Here's how the part is built. I have some questions about the finished solid (model axes, mm). Give positions to 0.01 mm unless a question says otherwise; leave off trailing zeros. Loops run counter-clockwise (first coordinate to the right, second up) from the corner with the lowest first, then second, coordinate; pieces in that order, holes last.
Q1. Suppose I cut it at A-A (z = 0). List the corners of the cut face in (x, y) for me (3 decimals), and give its area (3 significant figures).
Q2. Thinking about a two-plate mould opening in Y: for faces 1 (the face through (-7.559, 214.845, 5.796)), 2 (the face through (-4, 0, -4)), which applies, pulls with the +Y half, pulls with the -Y half, needs draft (parallel to the pull), parting line crosses it, or undercut?
Q3. I'm going to push flat-ended pins straight in: P1, Ø12.5, axis at x = 63.5, z = 285.75, coming from the +Y side; P2, Ø8.5, axis at x = -63.5, z = 285.75, coming from the -Y side. Where does each tip first touch, or does it pass through?
Q4. I need wall thicknesses on probe 1 along Z at (x, y) = (63.5, 2.25); probe 2 along Z at (x, y) = (-285.75, 3.25). Which ranges of each line are inside material? Lowest first, please.
Q5. Suppose I cut it at C-C (y = 148). List the corners of the cut face in (x, z) for me (3 decimals).
Q6. Suppose I cut it at B-B (x = 0). List the corners of the cut face in (y, z) for me (3 decimals), and give its area (3 significant figures).
Q7. Suppose I cut it at D-D (z = -262.5). List the corners of the cut face in (x, y) for me.
```python
from build123d import *

# Parameters (mm, degrees)
SKETCH1_W                        = 609.6
SKETCH1_H                        = 609.6
BOSS_EXTRUDE1_DEPTH              = 6.35
F_3_8_0_375_DIAMETER_HOLE1_D     = 9.525
F_3_8_0_375_DIAMETER_HOLE1_DEPTH = 11.684
F_3_8_0_375_DIAMETER_HOLE1_TIP   = 2.861598698
SKETCH4_R                        = 9.525
BOSS_EXTRUDE2_DEPTH              = 422.91


with BuildPart() as part:
    # Sketch1 → Boss-Extrude1 (new body)
    with BuildSketch(Plane(origin=(0, 0, 0), x_dir=(1, 0, 0), z_dir=(0, 1, 0))):
        Rectangle(SKETCH1_W, SKETCH1_H)
    extrude(amount=BOSS_EXTRUDE1_DEPTH)

    # 3/8 (0.375) Diameter Hole1
    with Locations(Plane(origin=(0, 6.35, 0), x_dir=(1, 0, 0), z_dir=(0, 1, 0))):
        with Locations((-63.5, -285.75), (63.5, -285.75), (-285.75, 63.5), (-285.75, -63.5), (-63.5, -180.975), (63.5, -180.975), (-180.975, -63.5), (-180.975, 63.5)):
            Hole(F_3_8_0_375_DIAMETER_HOLE1_D / 2, depth=F_3_8_0_375_DIAMETER_HOLE1_DEPTH)
            with Locations((0, 0, -(F_3_8_0_375_DIAMETER_HOLE1_DEPTH + F_3_8_0_375_DIAMETER_HOLE1_TIP / 2))):  # 118° drill point
                Cone(0, F_3_8_0_375_DIAMETER_HOLE1_D / 2, F_3_8_0_375_DIAMETER_HOLE1_TIP, mode=Mode.SUBTRACT)

    # Sketch4 → Boss-Extrude2 (add)
    with BuildSketch(Plane(origin=(0, 6.35, 0), x_dir=(1, 0, 0), z_dir=(0, 1, 0))):
        Circle(SKETCH4_R)
    extrude(amount=BOSS_EXTRUDE2_DEPTH)

    # Sketch5 → Revolve3 (revolve)
    with BuildSketch(Plane.XY):
        with BuildLine():
            Line((0, 457.835), (0, 426.085))
            ThreePointArc((0, 426.085), (-15.875, 441.96), (0, 457.835))
        make_face()
    revolve(axis=Axis((0, 599.823656089, 0), (0, -1, 0)))


solid = part.part
```
Solutions:
1. outline: (-304.8, 0) - (304.8, 0) - (304.8, 6.35) - (9.525, 6.35) - (9.525, 429.26) arc R15.875 ccw (long way) to (-9.525, 429.26) - (-9.525, 6.35) - (-304.8, 6.35) - close
1. area: 12,700 mm2
2. face 1: undercut
2. face 2: pulls with the -Y half
3. P1: stops at y = 6.35
3. P2: passes through
4. probe 1: z = -304.8 to 176.21, 185.74 to 280.99, 290.51 to 304.8
4. probe 2: z = -304.8 to -68.26, -58.74 to 58.74, 68.26 to 304.8
5. outline: circle Ø19.05 at (0, 0)
6. outline: (0, -304.8) - (6.35, -304.8) - (6.35, -9.525) - (429.26, -9.525) arc R15.875 ccw (long way) to (429.26, 9.525) - (6.35, 9.525) - (6.35, 304.8) - (0, 304.8) - close
6. area: 12,700 mm2
7. outline: (-304.8, 0) - (304.8, 0) - (304.8, 6.35) - (-304.8, 6.35) - close
